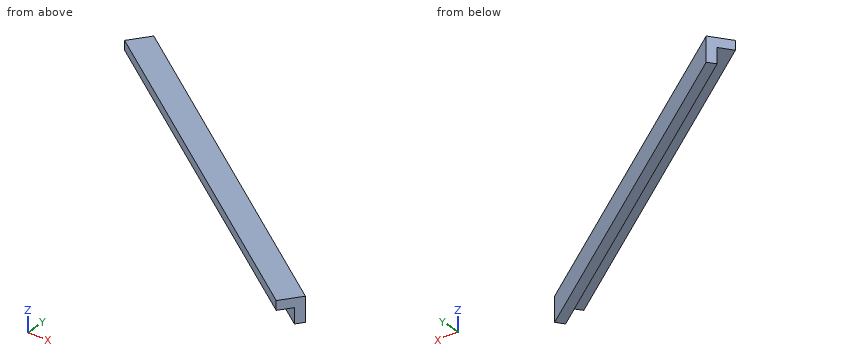
```python
from build123d import *

# Parameters (mm, degrees)
BOX127_W               = 0.8
BOX127_H               = 14
BOX127_DEPTH           = 0.8
BOX128_W               = 0.8
BOX128_H               = 14
BOX128_DEPTH           = 0.8
CUT067_PLACEMENT_ANGLE = 53


with BuildPart() as cubo127:
    # Box127 → Box127 (new body)
    with BuildSketch(Plane.XY):
        with Locations((0.4, 7)):
            Rectangle(BOX127_W, BOX127_H)
    extrude(amount=BOX127_DEPTH)


with BuildPart() as obj1:
    # Box128 → Box128 (new body)
    with BuildSketch(Plane(origin=(0.3, 0, 0.3), x_dir=(1, 0, 0), z_dir=(0, 0, 1))):
        with Locations((0.4, 7)):
            Rectangle(BOX128_W, BOX128_H)
    extrude(amount=BOX128_DEPTH)

    # Cut067: cut Cubo127
    add(cubo127.part, mode=Mode.SUBTRACT)


with BuildPart() as obj1_1:
    # Cut067 placement: moved
    add(obj1.part.moved(Location((-175.4, 133.4, -1.45))).rotate(Axis((-175.4, 133.4, -1.45), (0, 0, 1)), CUT067_PLACEMENT_ANGLE))


solid = obj1_1.part
```
CAD build for the part. Positions are in the model's coordinates, mm. Give positions to 0.01 mm unless a question says otherwise; leave off trailing zeros. Loops run counter-clockwise (first coordinate to the right, second up) from the corner with the lowest first, then second, coordinate; pieces in that order, holes last. Notation, with made-up numbers: M 43,-1.5 L 61,-1.5 A38 ccw 61,37.5 Z; hole C 72.25,-5 d7. An arc over 180 degrees is marked long. Use one line per item in the form item = value.
Item 1: Drill centre lines: probe 1 along Z at (x, y) = (-182, 139.25); probe 2 along X at (y, z) = (136.5, -0.7); probe 3 along X at (y, z) = (142.25, -0.5). Where is each one in solid material? Low to high. Write a range as from..to.
Determined:
probe_1 = -0.65..-0.35
probe_2 = -178.18..-177.69
probe_3 = -186.26..-185.32
Item 2: Slice it at C-C (x = -181). List the corners of the cut face in (y, z).
Determined:
outline = M 138,-0.65 L 138.62,-0.65 L 138.62,-1.15 L 139,-1.15 L 139,-0.35 L 138,-0.35 Z
Item 3: Slice it at A-A (z = -0.95). List the corners of the cut face in (x, y), plus the area to 3 significant figures.
Determined:
outline = M -186.1,142.46 L -174.92,134.04 L -174.74,134.28 L -185.92,142.7 Z
area = 4.20 mm2
Item 4: Slice it at B-B (y = 138.75). List the corners of the cut face in (x, z).
Determined:
outline = M -182,-0.65 L -181.17,-0.65 L -181.17,-1.15 L -180.67,-1.15 L -180.67,-0.35 L -182,-0.35 Z
